Build history of the part. All positions in model axes, mm. Face numbers are marked on the shaded views. Give positions to 0.01 mm unless a question says otherwise; leave off trailing zeros. Loops run counter-clockwise (first coordinate to the right, second up) from the corner with the lowest first, then second, coordinate; pieces in that order, holes last. Notation, with made-up numbers: (19, 5.5) -> (62, 5.5) arc R17 cw to (62, 13.5) -> close; hole circle Ø1 at (-26.5, -20). An arc over 180 degrees is marked (long way). Answer as a JSON object with one key per item and string values. Group by question number.
Q1. Wall check: probe 1 along Y at (x, z) = (-37.25, 1.2); probe 2 along Z at (x, y) = (-102, -6.5); probe 3 along X at (y, z) = (-3.5, 8). Give the ranges that are in metal, low to high. Write a range as from..to.
Q2. Two-plate mould, pull along Z, no slides. Class the marked faces 1, 2 and 3: pulls with the +Z half, pulls with the -Z half, needs draft (parallel to the pull), parting line crosses it, or undercut.
Q3. Band-saw the part on D-D, the plane z = 27.5. Write the cut outline in (x, y), plus the area to 4 significant figures.
Q4. Band-saw the part on C-C, the plane x = -37.25. Write the cut outline in (y, z), plus the area to 3 significant figures.
Q5. Drop flat-ended pins along their axis: pin 1 (4 mm diameter, centred on x = -21.25, y = 0, fed in from +Z); pin 2 (4 mm diameter, centred on x = -72, z = 5, fed in from -Y); pin 3 (6.5 mm diameter, centred on y = 0, z = 16.975, fed in from +X); pin 4 (1.3 mm diameter, centred on x = -71.5, z = 1, fed in from -Y). Give the stop position or say it passes through.
Q6. Band-saw the part on B-B, the plane y = -21.25. Write the cut outline in (x, z) (3 decimals), plus the area to 3 significant figures.
Q7. Band-saw the part on A-A, the plane y = 0. Count the separate pieces of the cut face and the enclosed holes in it, plus the area to 3 significant figures.
from build123d import *

# Parameters (mm, degrees)
BOSS_EXTRUDE1_DEPTH = 1.59
SKETCH2_W           = 1.59
SKETCH2_H           = 45
BOSS_EXTRUDE2_DEPTH = 32
SKETCH3_R           = 2.5
SKETCH3_R_2         = 1.75
CUT_EXTRUDE1_DEPTH  = 123.223711284
SKETCH4_R           = 2.5
SKETCH4_R_2         = 1.75
CUT_EXTRUDE2_DEPTH  = 138.687340377


with BuildPart() as part:
    # Sketch1 → Boss-Extrude1 (new body)
    with BuildSketch(Plane.XY):
        with BuildLine():
            Line((0, 16), (-114.34, 16))
            Line((-114.34, 16), (-114.34, -16))
            Line((-114.34, -16), (0, -16))
            ThreePointArc((0, -16), (16, 0), (0, 16))
        make_face()
    extrude(amount=BOSS_EXTRUDE1_DEPTH)

    # Sketch2 → Boss-Extrude2 (add)
    with BuildSketch(Plane.XY.offset(1.59)):
        with Locations((-113.545, -6.5)):
            Rectangle(SKETCH2_W, SKETCH2_H)
    extrude(amount=BOSS_EXTRUDE2_DEPTH)

    # Sketch3 → Cut-Extrude1 (cut, through all)
    with BuildSketch(Plane.XY.offset(1.59)):
        Circle(SKETCH3_R)
        with Locations((8.5, 0)):
            Circle(SKETCH3_R_2)
        with Locations((-21.25, 0)):
            Circle(SKETCH3_R_2)
        with Locations((-37.25, 0)):
            Circle(SKETCH3_R_2)
        with Locations((-67, 0)):
            Circle(SKETCH3_R_2)
        with Locations((-86.16, 0)):
            Circle(SKETCH3_R_2)
    extrude(amount=-CUT_EXTRUDE1_DEPTH, mode=Mode.SUBTRACT)

    # Sketch4 → Cut-Extrude2 (cut, through all)
    with BuildSketch(Plane.ZY.offset(114.34)):
        with Locations((16.975, 0)):
            Circle(SKETCH4_R)
        with Locations((16.975, 8.5)):
            Circle(SKETCH4_R_2)
        with Locations((16.975, -21.25)):
            Circle(SKETCH4_R_2)
    extrude(amount=-CUT_EXTRUDE2_DEPTH, mode=Mode.SUBTRACT)


solid = part.part
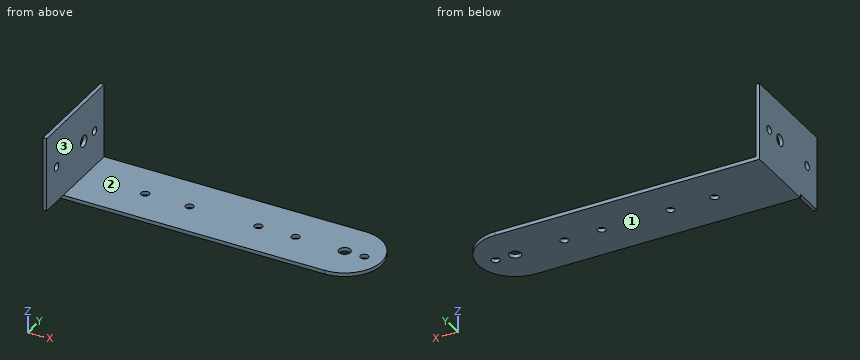
Worked answers:
{
 "1": {"probe 1": "-16..-1.75, 1.75..16", "probe 2": "0..1.59", "probe 3": "-114.34..-112.75"},
 "2": {"face 1": "pulls with the -Z half", "face 2": "pulls with the +Z half", "face 3": "needs draft"},
 "3": {"outline": "(-114.34, -29) -> (-112.75, -29) -> (-112.75, 16) -> (-114.34, 16) -> close", "area": "71.55 mm2"},
 "4": {"outline": "(-16, 0) -> (-1.75, 0) -> (-1.75, 1.59) -> (-16, 1.59) -> close; (1.75, 0) -> (16, 0) -> (16, 1.59) -> (1.75, 1.59) -> close", "area": "45.3 mm2"},
 "5": {"pin 1": "z = 1.59", "pin 2": "through", "pin 3": "x = -112.75", "pin 4": "y = -16"},
 "6": {"outline": "(-114.34, 1.59) -> (-112.75, 1.59) -> (-112.75, 15.225) -> (-114.34, 15.225) -> close; (-114.34, 18.725) -> (-112.75, 18.725) -> (-112.75, 33.59) -> (-114.34, 33.59) -> close", "area": "45.3 mm2"},
 "7": {"separate pieces": "8", "enclosed holes": "0", "area": "214 mm2"}
}
